Can you work these out from the model? Positions are in its coordinate system, mm. Face numbers are marked on the shaded views. A direction names the side the tool comes from. Give positions to 0.01 mm unless a question says otherwise; leave off trailing zeros. Write each loop counter-clockwise with the first axis right and the second up, starting at its lowest first coordinate (ties: lowest second). Pieces come first, ordered by that corner, then holes.
1. Suppose I cut it at C-C (y = 3.75). Please give me the cut outline in (x, z) (1 decimal), and give its area (3 significant figures).
2. Suppose I cut it at B-B (z = 0). Please give me the cut outline in (x, y), and give its area (3 significant figures).
3. Suppose I cut it at A-A (x = 0). Please give me the cut outline in (y, z).
4. If I drill on probe 1 along Y at (x, z) = (-1.5, 4.25); probe 2 along Y at (x, z) = (-0.25, -3); probe 3 along Y at (x, z) = (2.5, -0.75), over which ranges is the centre line in solid material (lowest first)?
5. On a 3-axis mill with a long thin cutter (end or side, diameter ignored), from which of +Z, -Z, +X, -X, +Y, -Y can I reach the whole of each face in a straight line? I mean the marked faces 1, 2 and 3. Say none if no direction works.
6. Suppose I cut it at D-D (y = 11.5). Please give me the cut outline in (x, z).
7. I'm going to push flat-ended pins straight in: pin 1 (1 mm diameter, centred on x = 0.5, y = 8.5, fed in from -Z); pin 2 (1 mm diameter, centred on x = 1.5, z = -3, fed in from +Y). Where does each tip first touch, or does it pass through?
```python
from build123d import *

# Parameters (mm, degrees)
FILLET1_R     = 0.127
CHAMFER1_SIZE = 0.508


with BuildPart() as part:
    # Sketch1 → Revolve1 (revolve)
    with BuildSketch(Plane.XY):
        with BuildLine():
            Line((0, 23.368), (3.17119, 23.368))
            Line((3.17119, 23.368), (3.17119, 5.334))
            ThreePointArc((3.17119, 5.334), (2.774555586, 4.826), (3.17119, 4.318))
            Line((3.17119, 4.318), (4.7625, 4.318))
            Line((4.7625, 4.318), (4.7625, 1.778))
            Line((4.7625, 1.778), (2.3749, 1.778))
            Line((2.3749, 1.778), (2.3749, 0))
            Line((2.3749, 0), (0, 0))
            Line((0, 0), (0, 23.368))
        make_face()
    revolve(axis=Axis((0, 0, 0), (0, 1, 0)))

    # Fillet1
    fillet1_edges = [part.edges().sort_by_distance(p)[0] for p in [
        (-2.3749, 1.778, 0),
    ]]
    fillet(fillet1_edges, radius=FILLET1_R)

    # Chamfer1
    chamfer1_edges = [part.edges().sort_by_distance(p)[0] for p in [
        (-3.17119, 23.368, 0),
    ]]
    chamfer(chamfer1_edges, length=CHAMFER1_SIZE)


solid = part.part
```
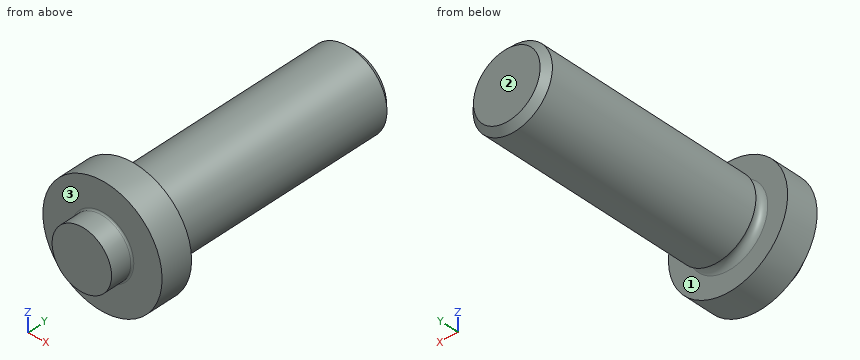
Checks:
1. outline: circle Ø9.5 at (0, 0)
1. area: 71.3 mm2
2. outline: (-4.76, 1.78) - (-2.5, 1.78) arc R0.13 cw to (-2.37, 1.65) - (-2.37, 0) - (2.37, 0) - (2.37, 1.65) arc R0.13 cw to (2.5, 1.78) - (4.76, 1.78) - (4.76, 4.32) - (3.17, 4.32) arc R0.52 cw to (3.17, 5.33) - (3.17, 22.86) - (2.66, 23.37) - (-2.66, 23.37) - (-3.17, 22.86) - (-3.17, 5.33) arc R0.52 cw to (-3.17, 4.32) - (-4.76, 4.32) - close
2. area: 153 mm2
3. outline: (0, -2.37) - (1.65, -2.37) arc R0.13 cw to (1.78, -2.5) - (1.78, -4.76) - (4.32, -4.76) - (4.32, -3.17) arc R0.52 cw to (5.33, -3.17) - (22.86, -3.17) - (23.37, -2.66) - (23.37, 2.66) - (22.86, 3.17) - (5.33, 3.17) arc R0.52 cw to (4.32, 3.17) - (4.32, 4.76) - (1.78, 4.76) - (1.78, 2.5) arc R0.13 cw to (1.65, 2.37) - (0, 2.37) - close
4. probe 1: y = 1.78 to 4.32
4. probe 2: y = 1.78 to 4.39, 5.26 to 23.02
4. probe 3: y = 1.78 to 23.37
5. face 1: +Y
5. face 2: +Z, -Z, +X, -X, +Y
5. face 3: -Y
6. outline: circle Ø6.34 at (0, 0)
7. pin 1: stops at z = -3.17
7. pin 2: stops at y = 23.18
